from build123d import *

# Parameters (mm, degrees)
SKETCH1_W           = 52.1
SKETCH1_H           = 14
BOSS_EXTRUDE1_DEPTH = 4
SKETCH2_W           = 57.5
SKETCH2_H           = 90
BOSS_EXTRUDE2_DEPTH = 4
SKETCH3_R           = 1.5
BOSS_EXTRUDE3_DEPTH = 2.8
SKETCH4_R           = 1.5
BOSS_EXTRUDE4_DEPTH = 2.8


with BuildPart() as part:
    # Sketch1 → Boss-Extrude1 (new body)
    with BuildSketch(Plane.XY.offset(18.5)):
        with Locations((-100.65, 0)):
            Rectangle(SKETCH1_W, SKETCH1_H)
    extrude(amount=BOSS_EXTRUDE1_DEPTH)

    # Sketch2 → Boss-Extrude2 (add)
    with BuildSketch(Plane(origin=(-126.7, 0, 0), x_dir=(0, 0, -1), z_dir=(1, 0, 0))):
        with Locations((6.25, 0)):
            Rectangle(SKETCH2_W, SKETCH2_H)
    extrude(amount=BOSS_EXTRUDE2_DEPTH)

    # Sketch3 → Boss-Extrude3 (add)
    with BuildSketch(Plane.XY.offset(15.7)):
        with Locations((-89.6, 4)):
            Circle(SKETCH3_R)
        with Locations((-89.6, -4)):
            Circle(SKETCH3_R)
        with Locations((-97.6, 4)):
            Circle(SKETCH3_R)
        with Locations((-97.6, -4)):
            Circle(SKETCH3_R)
    extrude(amount=BOSS_EXTRUDE3_DEPTH)

    # Sketch4 → Boss-Extrude4 (add)
    with BuildSketch(Plane(origin=(-129.5, 0, 0), x_dir=(0, 0, -1), z_dir=(1, 0, 0))):
        with Locations((15, -30)):
            Circle(SKETCH4_R)
        with Locations((-15, -30)):
            Circle(SKETCH4_R)
        with Locations((15, 30)):
            Circle(SKETCH4_R)
        with Locations((-15, 30)):
            Circle(SKETCH4_R)
    extrude(amount=BOSS_EXTRUDE4_DEPTH)


solid = part.part
Read the model definition and answer for the solid it produces. Units are mm, in the model's axes. A direction names the side the tool comes from. Give positions to 0.01 mm unless a question says otherwise; leave off trailing zeros. Loops run counter-clockwise (first coordinate to the right, second up) from the corner with the lowest first, then second, coordinate; pieces in that order, holes last. Notation, with made-up numbers: (78.25, 20.5) - (123.25, 20.5) arc R19 cw to (123.25, 55.5) - close; hole circle Ø10 at (55.5, 27). An arc over 180 degrees is marked (long way). Answer as CSV lines item,"result". Start each with the question number.
1) Which of the six approach directions +Z, -Z, +X, -X, +Y, -Y give full straight-line access (tool end or side, diameter ignored) to faces 1 (the face through (-99, 7, 20)), 2 (the face through (-91.1, 4.07, 17.08)), 3 (the face through (-98, -4, 15.7)), 4 (the face through (-128.12, -28.99, -13.89))?
2) Find section B-B (x = -97.6). Write down the section's boundary in (y, z), then the cut area to 3 significant figures.
3) Straight lines are drawn through the part: L1, parallel to X at y = 25, z = -6; L2, parallel to Z at x = -113, y = 2. For each, find the intervals that lie inside material, in ascending order. Write a range as from..to.
4) Find section C-C (z = -4.5). Write down the section's boundary in (x, y), then the cut area to 3 significant figures.
5) Find section A-A (y = -30). Write down the section's boundary in (x, z).
6) Determine the mould class of faces 5 (the face through (-99, -7, 20)), 6 (the face through (-91.1, -3.93, 17.08)), 7 (the face through (-129.5, -30, 15)) for opening direction X: released by +X, released by -X, zero draft, split by the parting line, or undercut.
7) Each of these flat-tipped pins is pushed along its axis until it touches: pin 1 Ø5 at (y, z) = (-22.5, 4.5) entering from -X; pin 2 Ø3 at (x, z) = (-88.5, 21) entering from -Y; pin 3 Ø1 at (y, z) = (17.5, -15) entering from +X. Where does it stop, or does it pass through?
8) Find section D-D (y = -4). Write down the section's boundary in (x, z).
Findings below:
1,face 1,"+Z, -Z, +X, +Y"
1,face 2,"-Z"
1,face 3,"-Z, +X, +Y, -Y"
1,face 4,"-X"
2,outline,"(-7, 18.5) - (-5.5, 18.5) - (-5.5, 15.7) - (-2.5, 15.7) - (-2.5, 18.5) - (2.5, 18.5) - (2.5, 15.7) - (5.5, 15.7) - (5.5, 18.5) - (7, 18.5) - (7, 22.5) - (-7, 22.5) - close"
2,area,"72.8 mm^2"
3,L1,"-126.7..-122.7"
3,L2,"18.5..22.5"
4,outline,"(-126.7, -45) - (-122.7, -45) - (-122.7, 45) - (-126.7, 45) - close"
4,area,"360 mm^2"
5,outline,"(-129.5, -16.5) - (-126.7, -16.5) - (-126.7, -35) - (-122.7, -35) - (-122.7, 22.5) - (-126.7, 22.5) - (-126.7, 16.5) - (-129.5, 16.5) - (-129.5, 13.5) - (-126.7, 13.5) - (-126.7, -13.5) - (-129.5, -13.5) - close"
6,face 5,"zero draft"
6,face 6,"undercut"
6,face 7,"released by -X"
7,pin 1,"x = -126.7"
7,pin 2,"y = -7"
7,pin 3,"x = -122.7"
8,outline,"(-126.7, -35) - (-122.7, -35) - (-122.7, 18.5) - (-99.1, 18.5) - (-99.1, 15.7) - (-96.1, 15.7) - (-96.1, 18.5) - (-91.1, 18.5) - (-91.1, 15.7) - (-88.1, 15.7) - (-88.1, 18.5) - (-74.6, 18.5) - (-74.6, 22.5) - (-126.7, 22.5) - close"
